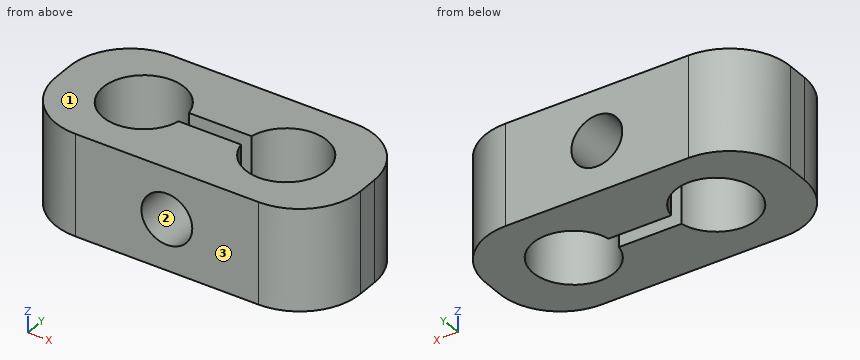
Autodesk Inventor part; units mm, degrees
ref_plane "YZ Plane" through (0, 0, 0) normal (1, 0, 0) x (0, 1, 0)
ref_plane "XZ Plane" through (0, 0, 0) normal (0, 1, 0) x (-1, 0, 0)
ref_plane "XY Plane" through (0, 0, 0) normal (0, 0, 1) x (1, 0, 0)
sketch "Sketch1" plane through (0, 0, 0) normal (0, 0, 1) x (1, 0, 0)
  line L0 (0, 0) -> (-14, 0) construction
  circle A0 centre (-14, 0) radius 4
  circle A1 centre (0, 0) radius 4
  line L1 (8, -7) -> (-22, -7)
  line L2 (-22, -7) -> (-22, 7)
  line L3 (-22, 7) -> (8, 7)
  line L4 (8, 7) -> (8, -7)
  line L5 (8, -7) -> (-22, 7) construction
  line L6 (-22, -7) -> (8, 7) construction
  point P0 (-7, 0)
  dimension "d0" = 8
  dimension "d1" = 14
  dimension "d2" = 8
  dimension "d3" = 14
  dimension "d13" = 30
extrude "Extrusion1" add sketch "Sketch1" along normal blind 10
sketch "Sketch2" plane through (-22, 7, 0) normal (0, 1, 0) x (1, 0, 0)
  line L0 (0, 0) -> (30, 0)
  line L1 (30, -10) -> (0, -10)
  line L2 (15, 0) -> (15, -10) construction
  circle A0 centre (15, -5) radius 2.5
  point P0 (22, 0)
  dimension "d6" = 5
extrude "Extrusion2" cut sketch "Sketch2" against normal through all
fillet "Fillet1" radius 6 4 edges at (8, 7, 5) (-22, 7, 5) (-22, -7, 5) (8, -7, 5)
sketch "Sketch3" plane through (0, 0, 10) normal (0, 0, 1) x (1, 0, 0)
  line L0 (-16, -7) -> (2, -7)
  circle A0 centre (0, 0) radius 4
  circle A1 centre (-14, 0) radius 4
  line L1 (-14, 0) -> (0, 0) construction
  line L2 (0, -0.75) -> (-14, -0.75)
  line L3 (-14, -0.75) -> (-14, 0.75)
  line L4 (-14, 0.75) -> (0, 0.75)
  line L5 (0, 0.75) -> (0, -0.75)
  line L6 (0, -0.75) -> (-14, 0.75) construction
  line L7 (-14, -0.75) -> (0, 0.75) construction
  point P0 (-7, 0)
  dimension "d10" = 1.5
extrude "Extrusion3" cut sketch "Sketch3" against normal through all contours L4 L5 L2 A0 | A0 L2 A1 L4 | A1 L2 L3 L4 picked at (-1.3307, -0.0838) picked at (-12.6667, 0)
properties part number "crank web"
CAD build for the part. Positions are in the model's coordinates, mm. Face numbers are marked on the shaded views. Round coordinates to 2 decimals unless told otherwise and drop trailing zeros. Write each loop counter-clockwise with the first axis right and the second up, starting at its lowest first coordinate (ties: lowest second). Pieces come first, ordered by that corner, then holes. Notation, with made-up numbers: (25, -17) - (53, -17) arc R24 cw to (53, 14) - close; hole circle Ø5 at (46, 53). An arc over 180 degrees is marked (long way). Return JSON: item names as keys, results as strings. Group by question number.
Item 1: Probe probe 1 along Z at (x, y) = (-7, 3.25); probe 2 along X at (y, z) = (-1.75, 2.25); probe 3 along Y at (x, z) = (0, 7.75). List the from-to ranges inside material, lowest first.
Item 2: Mould opens along Z. For the marked faces 1, 2 and 3 say: +Z half, -Z half, draft (parallel to the pull), parting line (faces both ways), or undercut.
Item 3: Band-saw the part on B-B on y = 0. List the corners of the cut face in (x, z), plus the area to 3 significant figures.
Item 4: Band-saw the part on C-C on z = 9. List the corners of the cut face in (x, y), plus the area to 3 significant figures.
Item 5: Band-saw the part on A-A on x = 0. List the corners of the cut face in (y, z).
Item 6: Band-saw the part on D-D on y = 1.5. List the corners of the cut face in (x, z).
Item 7: Flat gauge pins, fed straight in: pin 1 Ø1.5 at (x, z) = (-17, 5) entering from +Y; pin 2 Ø1 at (y, z) = (-5, 2) entering from -X; pin 3 Ø4 at (y, z) = (-5.5, 5) entering from +X. Where does each tip first touch, or does it go through?
Resolved:
{
 "1": {"probe 1": "z = 0 to 2.5, 7.5 to 10", "probe 2": "x = -21.95 to -17.6, -10.4 to -3.6, 3.6 to 7.95", "probe 3": "y = -7 to -4, 4 to 7"},
 "2": {"face 1": "+Z half", "face 2": "undercut", "face 3": "draft"},
 "3": {"outline": "(-22, 0) - (-18, 0) - (-18, 10) - (-22, 10) - close; (4, 0) - (8, 0) - (8, 10) - (4, 10) - close", "area": "80.0 mm²"},
 "4": {"outline": "(-22, -1) arc R6 ccw to (-16, -7) - (2, -7) arc R6 ccw to (8, -1) - (8, 1) arc R6 ccw to (2, 7) - (-16, 7) arc R6 ccw to (-22, 1) - close; hole (-10.07, -0.75) - (-3.93, -0.75) arc R4 ccw (long way) to (-3.93, 0.75) - (-10.07, 0.75) arc R4 ccw (long way) to start", "area": "279 mm²"},
 "5": {"outline": "(-7, 0) - (-4, 0) - (-4, 10) - (-7, 10) - close; (4, 0) - (7, 0) - (7, 10) - (4, 10) - close"},
 "6": {"outline": "(-21.98, 0) - (-17.71, 0) - (-17.71, 10) - (-21.98, 10) - close; (-10.29, 0) - (-3.71, 0) - (-3.71, 10) - (-10.29, 10) - close; (3.71, 0) - (7.98, 0) - (7.98, 10) - (3.71, 10) - close; hole circle Ø5 at (-7, 5)"},
 "7": {"pin 1": "stops at y = 6.99", "pin 2": "stops at x = -20.87", "pin 3": "stops at x = 7.45"}
}
